```python
from build123d import *

# Parameters (mm, degrees)
SKETCH1_R               = 4
BOSS_EXTRUDE1_DEPTH     = 6
SKETCH2_R               = 2.75
CUT_EXTRUDE1_DEPTH      = 6
SKETCH3_R               = 4
BOSS_EXTRUDE2_DEPTH     = 2
SKETCH4_R               = 1
CUT_EXTRUDE2_DEPTH      = 2
SKETCH9_W               = 4
SKETCH9_H               = 3.175
CUT_EXTRUDE8_DEPTH      = 2
CUT_EXTRUDE8_DEPTH_BACK = 2


with BuildPart() as part:
    # Sketch1 → Boss-Extrude1 (new body)
    with BuildSketch(Plane.XY):
        Circle(SKETCH1_R)
    extrude(amount=-BOSS_EXTRUDE1_DEPTH)

    # Sketch2 → Cut-Extrude1 (cut)
    with BuildSketch(Plane(origin=(0, 0, -6), x_dir=(-1, 0, 0), z_dir=(0, 0, -1))):
        Circle(SKETCH2_R)
    extrude(amount=-CUT_EXTRUDE1_DEPTH, mode=Mode.SUBTRACT)

    # Sketch3 → Boss-Extrude2 (add)
    with BuildSketch(Plane(origin=(0, 0, -6), x_dir=(-1, 0, 0), z_dir=(0, 0, -1))):
        Circle(SKETCH3_R)
    extrude(amount=BOSS_EXTRUDE2_DEPTH)

    # Sketch4 → Cut-Extrude2 (cut)
    with BuildSketch(Plane(origin=(0, 0, -8), x_dir=(-1, 0, 0), z_dir=(0, 0, -1))):
        Circle(SKETCH4_R)
    extrude(amount=-CUT_EXTRUDE2_DEPTH, mode=Mode.SUBTRACT)

    # Sketch9 → Cut-Extrude8 (cut, two sides)
    with BuildSketch(Plane(origin=(3.998726485, 0, 0), x_dir=(0, 0, -1), z_dir=(1, 0, 0))) as cut_extrude8_sk:
        with Locations((5.25, 0.9125)):
            Rectangle(SKETCH9_W, SKETCH9_H)
    extrude(amount=CUT_EXTRUDE8_DEPTH, mode=Mode.SUBTRACT)
    extrude(cut_extrude8_sk.sketch, amount=-CUT_EXTRUDE8_DEPTH_BACK, mode=Mode.SUBTRACT)


solid = part.part
```
Build history of the part. All positions in model axes, mm. A direction names the side the tool comes from. Round coordinates to 2 decimals unless told otherwise and drop trailing zeros. Write each loop counter-clockwise with the first axis right and the second up, starting at its lowest first coordinate (ties: lowest second). Pieces come first, ordered by that corner, then holes.
1) Mould opens along Y. For faces 4 (the flat face through (-1.2, 0, -6)), 5 (the flat face through (-1, -1, -8)) say: +Y half, -Y half, draft (parallel to the pull), parting line (faces both ways), or undercut.
2) Pin check, flat tips, straight feed: pin 1 (1 mm diameter, centred on x = 3.5, z = -5.5, fed in from +Y); pin 2 (0.9 mm diameter, centred on x = 2.5, z = -5.5, fed in from -Y); pin 3 (1 mm diameter, centred on y = 0.5, z = -4.5, fed in from +X). Stop position of each tip, or through.
3) Drill centre lines: probe 1 along Y at (x, z) = (0, -7.25); probe 2 along Z at (x, y) = (3, 1.25); probe 3 along Y at (x, z) = (0, -4.5). Where is each one in solid material? Low to high.
4) Band-saw the part on B-B, the plane z = -6.25. List the corners of the cut face in (x, y) (1 decimal).
5) Band-saw the part on D-D, the plane y = -2.5. List the corners of the cut face in (x, z).
6) Band-saw the part on A-A, the plane x = 0. List the corners of the cut face in (y, z), and give its area (3 significant figures).
7) 3-axis set-ups, long thin cutter, end or side, ignore diameter. For faces 1 (the cylindrical face through (-2.54, -1.05, -3.04)), 2 (the flat face through (2.6, 2.5, -5.2)), 3 (the flat face through (3, 1, 0)): which of +Z, -Z, +X, -X, +Y, -Y reach the whole face in a straight line?
8) Band-saw the part on C-C, the plane y = 1.25. List the corners of the cut face in (x, z).
Ans:
1. face 4: undercut
1. face 5: draft
2. pin 1: stops at y = 2.65
2. pin 2: stops at y = -3.43
2. pin 3: stops at x = -2.56
3. probe 1: y = -4 to -1, 1 to 4
3. probe 2: z = -8 to -7.25, -3.25 to 0
3. probe 3: y = -4 to -2.75, 2.75 to 4
4. outline: (2, -0.7) - (2, 2.5) - (3.1, 2.5) arc R4 ccw (long way) to (3.9, -0.7) - close; hole circle Ø2 at (0, 0)
5. outline: (-3.12, -8) - (3.12, -8) - (3.12, 0) - (1.15, 0) - (1.15, -6) - (-1.15, -6) - (-1.15, 0) - (-3.12, 0) - close
6. outline: (-4, -8) - (-1, -8) - (-1, -6) - (-2.75, -6) - (-2.75, 0) - (-4, 0) - close; (1, -8) - (4, -8) - (4, 0) - (2.75, 0) - (2.75, -6) - (1, -6) - close
6. area: 27.0 mm2
7. face 1: +Z
7. face 2: +X
7. face 3: +Z, +X, -X, +Y, -Y
8. outline: (-3.8, -8) - (3.8, -8) - (3.8, -7.25) - (2, -7.25) - (2, -6) - (-2.45, -6) - (-2.45, 0) - (-3.8, 0) - close; (2.45, -3.25) - (3.8, -3.25) - (3.8, 0) - (2.45, 0) - close
